from build123d import *

# Parameters (mm, degrees)
F0_R     = 1.1
F1_DEPTH = 1.5
F2_R     = 1.1
F3_DEPTH = 1.5


with BuildPart() as f1:
    # F0 (on Top) → F1 (new body)
    with BuildSketch(Plane.XY):
        with BuildLine():
            Line((9.22254, 33), (-9.22254, 33))
            Line((-9.22254, 33), (-9.22254, -33))
            Line((-9.22254, -33), (-4, -33))
            Line((-4, -33), (-4, -30))
            ThreePointArc((-4, -30), (0, -26), (4, -30))
            Line((4, -30), (4, -33))
            Line((4, -33), (9.22254, -33))
            Line((9.22254, -33), (9.22254, 19.77746))
            Line((9.22254, 19.77746), (6.22254, 19.77746))
            ThreePointArc((6.22254, 19.77746), (2.22254, 23.77746), (6.22254, 27.77746))
            Line((6.22254, 27.77746), (9.22254, 27.77746))
            Line((9.22254, 27.77746), (9.22254, 33))
        make_face()
        with Locations((-6.22254, -30)):
            Circle(F0_R, mode=Mode.SUBTRACT)
        with Locations((-4.4, -25.6)):
            Circle(F0_R, mode=Mode.SUBTRACT)
        with Locations((4.4, -25.6)):
            Circle(F0_R, mode=Mode.SUBTRACT)
        with Locations((0, -23.77746)):
            Circle(F0_R, mode=Mode.SUBTRACT)
        with Locations((6.22254, -30)):
            Circle(F0_R, mode=Mode.SUBTRACT)
        with Locations((1.82254, 19.37746)):
            Circle(F0_R, mode=Mode.SUBTRACT)
        with Locations((0, 23.77746)):
            Circle(F0_R, mode=Mode.SUBTRACT)
        with Locations((1.82254, 28.17746)):
            Circle(F0_R, mode=Mode.SUBTRACT)
        with Locations((6.22254, 17.554921)):
            Circle(F0_R, mode=Mode.SUBTRACT)
        with Locations((6.22254, 30)):
            Circle(F0_R, mode=Mode.SUBTRACT)
    extrude(amount=F1_DEPTH)

    # F2 (on face) → F3 (cut, through all)
    with BuildSketch(Plane.XY.offset(1.5)):
        with BuildLine():
            Line((-9.22254, 0), (9.22254, 0))
            Line((9.22254, 0), (9.22254, 19.77746))
            Line((9.22254, 19.77746), (6.22254, 19.77746))
            ThreePointArc((6.22254, 19.77746), (2.22254, 23.77746), (6.22254, 27.77746))
            Line((6.22254, 27.77746), (9.22254, 27.77746))
            Line((9.22254, 27.77746), (9.22254, 33))
            Line((9.22254, 33), (-9.22254, 33))
            Line((-9.22254, 33), (-9.22254, 0))
        make_face()
        with Locations((1.82254, 19.37746)):
            Circle(F2_R, mode=Mode.SUBTRACT)
        with Locations((0, 23.77746)):
            Circle(F2_R, mode=Mode.SUBTRACT)
        with Locations((1.82254, 28.17746)):
            Circle(F2_R, mode=Mode.SUBTRACT)
        with Locations((6.22254, 17.554921)):
            Circle(F2_R, mode=Mode.SUBTRACT)
        with Locations((6.22254, 30)):
            Circle(F2_R, mode=Mode.SUBTRACT)
    extrude(amount=-F3_DEPTH, mode=Mode.SUBTRACT)

    # F4: F1 across plane


with BuildPart() as f1_1:
    add(f1.part)
    add(f1.part.mirror(Plane.XZ))


solid = f1_1.part
The listing builds one solid part. Answer for the finished solid, in the listing's coordinates (mm). A direction names the side the tool comes from. Give positions to 0.01 mm unless a question says otherwise; leave off trailing zeros. Loops run counter-clockwise (first coordinate to the right, second up) from the corner with the lowest first, then second, coordinate; pieces in that order, holes last. Notation, with made-up numbers: (-8, 12.5) - (34, 12.5) arc R6 cw to (34, 20.5) - close; hole circle Ø2 at (8.25, 82.5). An arc over 180 degrees is marked (long way). Write each question's results on one line, items separated by ' | '.
1. Consider probe 1 along Y at (x, z) = (-4.4, 0.8); probe 2 along X at (y, z) = (30, 0.7); probe 3 along X at (y, z) = (-28.5, 1.25). Determine where each line is inside the solid, lowest interval first. Write a range as from..to.
Resolved:
probe 1: y = -33..-26.7, -24.5..24.5, 26.7..33 | probe 2: x = -9.22..-7.32, -5.12..-4, 4..5.12, 7.32..9.22 | probe 3: x = -9.22..-3.71, 3.71..9.22
2. Find section A-A, the plane x = 0. Write down the section's boundary in (y, z), then the cut area to 3 significant figures.
Resolved:
outline: (-26, 0) - (-24.88, 0) - (-24.88, 1.5) - (-26, 1.5) - close; (-22.68, 0) - (22.68, 0) - (22.68, 1.5) - (-22.68, 1.5) - close; (24.88, 0) - (26, 0) - (26, 1.5) - (24.88, 1.5) - close | area: 71.4 mm^2
3. Which of the six approach directions +Z, -Z, +X, -X, +Y, -Y give full straight-line access (tool end or side, diameter ignored) to faces 1 (the face through (6.73, -30.976, 0.74)), 2 (the face through (-4, 32, 1)), 3 (the face through (4, -31, 1))?
Resolved:
face 1: +Z, -Z | face 2: +Z, -Z, +Y | face 3: +Z, -Z, -Y
4. Find section C-C, the plane x = -2.75. Write down the section's boundary in (y, z), then the cut area to 3 significant figures.
Resolved:
outline: (-27.1, 0) - (27.1, 0) - (27.1, 1.5) - (-27.1, 1.5) - close | area: 81.3 mm^2
5. Find section B-B, the plane z = 0.65. Count the separate pieces of the cut face and the enclosed holes in it, then the cut area to 3 significant figures.
Resolved:
separate pieces: 1 | enclosed holes: 10 | area: 1,080 mm^2
6. A flat-ended cylindrical pin translates along its axis: P1, Ø1.3, axis at x = 0, y = 23.78, coming from the -Z side. Find the tip coordinate at first contact, or state that the pin passes through.
Resolved:
P1: passes through
7. For a pull along X with two mould halves and no side action, classify faces 4 (the face through (-0.24, 24.85, 0.74)), 5 (the face through (9.223, 0, 1)), 6 (the face through (0, 0, 1.5)) as +X half, -X half, draft (parallel to the pull), parting line (faces both ways), or undercut.
Resolved:
face 4: undercut | face 5: +X half | face 6: draft
